The listing builds one solid part. Answer for the finished solid, in the listing's coordinates (mm). A direction names the side the tool comes from. Round coordinates to 2 decimals unless told otherwise and drop trailing zeros. Loops run counter-clockwise (first coordinate to the right, second up) from the corner with the lowest first, then second, coordinate; pieces in that order, holes last. Notation, with made-up numbers: (12, -19) - (69, -19) arc R3 ccw to (69, -15) - close; hole circle Ø2 at (89.5, 1). An arc over 180 degrees is marked (long way). One line per item, written item: value.
```python
from build123d import *

# Parameters (mm, degrees)
BOSS_EXTRUDE1_DEPTH = 5
FILLET1_R           = 0.5


with BuildPart() as part:
    # Sketch1 → Boss-Extrude1 (new body)
    with BuildSketch(Plane.XY):
        with BuildLine():
            Line((-58.035421321, -29.898049549), (-52.781533871, -38.998049549))
            Line((-52.781533871, -38.998049549), (-47.781533871, -38.998049549))
            Line((-47.781533871, -38.998049549), (-50.93623441, -40.998049549))
            Line((-50.93623441, -40.998049549), (-53.93623441, -40.998049549))
            Line((-53.93623441, -40.998049549), (-59.767472129, -30.898049549))
            ThreePointArc((-59.767472129, -30.898049549), (-61.401962202, -24.798049549), (-59.767472129, -18.698049549))
            Line((-59.767472129, -18.698049549), (-53.93623441, -8.598049549))
            Line((-53.93623441, -8.598049549), (-51.291363981, -8.598049549))
            ThreePointArc((-51.291363981, -8.598049549), (-48.766460182, -4.985563469), (-44.583160049, -3.598049549))
            Line((-44.583160049, -3.598049549), (-44.583160049, -5.598049549))
            ThreePointArc((-44.583160049, -5.598049549), (-48.118693955, -7.062515643), (-49.583160049, -10.598049549))
            Line((-49.583160049, -10.598049549), (-52.781533871, -10.598049549))
            Line((-52.781533871, -10.598049549), (-58.035421321, -19.698049549))
            ThreePointArc((-58.035421321, -19.698049549), (-59.401962202, -24.798049549), (-58.035421321, -29.898049549))
        make_face()
    boss_extrude1 = extrude(amount=BOSS_EXTRUDE1_DEPTH)

    # Mirror1: Boss-Extrude1 across plane
    add(boss_extrude1.mirror(Plane(origin=(-44.583160049, -5.598049549, 5), x_dir=(0, 0, 1), z_dir=(-1, 0, 0))))

    # Fillet1
    fillet1_edges = [part.edges().sort_by_distance(p)[0] for p in [
        (-47.781533871, -38.998049549, 2.5),
        (-50.93623441, -40.998049549, 2.5),
        (-53.93623441, -40.998049549, 2.5),
        (-53.93623441, -8.598049549, 2.5),
        (-51.291363981, -8.598049549, 2.5),
        (-41.384786226, -38.998049549, 2.5),
        (-38.230085688, -40.998049549, 2.5),
        (-35.230085688, -40.998049549, 2.5),
        (-35.230085688, -8.598049549, 2.5),
        (-37.874956116, -8.598049549, 2.5),
    ]]
    fillet(fillet1_edges, radius=FILLET1_R)


solid = part.part
```
1) Each of these flat-tipped pins is pushed along its axis until it touches: pin 1 Ø10 at (x, y) = (-48, -28.5) entering from -Z; pin 2 Ø3 at (y, z) = (-30.5, 4) entering from +X; pin 3 Ø2 at (x, z) = (-35.5, 3.5) entering from +Y; pin 4 Ø2 at (y, z) = (-33, 1.5) entering from +X. Where does it stop, or does it pass through?
Final values:
pin 1: through
pin 2: x = -28.51
pin 3: y = -8.6
pin 4: x = -30.04
2) For faces 1 (the flat face through (-53, -8.598, 2)), 2 (the flat face through (-50.01, -40.41, 2.46)), 3 (the flat face through (-33.795, -15.084, 2.465)), determine the directions among +Z, -Z, +X, -X, +Y, -Y from which every point of the face is accessible in a straight line to the end or side of a thin tool.
Final values:
face 1: +Z, -Z, -X, +Y
face 2: +Z, -Z, -Y
face 3: +Z, -Z
3) A cutting plane is placed at A-A on y = -27. Give the vertices of the cut face in (x, z).
Final values:
outline: (-61.2, 0) - (-59.16, 0) - (-59.16, 5) - (-61.2, 5) - close; (-30, 0) - (-27.96, 0) - (-27.96, 5) - (-30, 5) - close
4) A cutting plane is placed at B-B on x = -33. Give the vertices of the cut face in (y, z).
Final values:
outline: (-37.14, 0) - (-33.14, 0) - (-33.14, 5) - (-37.14, 5) - close; (-16.46, 0) - (-12.46, 0) - (-12.46, 5) - (-16.46, 5) - close
5) Consider L1, parallel to X at y = -25, z = 4.35; L2, parallel to Y at x = -52.5, z = 2.6; L3, parallel to X at y = -37, z = 3. Determine where each line is inside the solid, lowest interval first.
Final values:
L1: -61.4 to -59.4, -29.77 to -27.77
L2: -41 to -39, -10.6 to -8.6
L3: -56.24 to -53.94, -35.23 to -32.92
6) A cutting plane is placed at C-C on x = -47. Give the vertices of the cut face in (y, z), and give its area (3 significant figures).
Final values:
outline: (-6.22, 0) - (-4.03, 0) - (-4.03, 5) - (-6.22, 5) - close
area: 11.0 mm2
7) For a pull along X with two mould halves and no side action, classify faces 4 (the flat face through (-37, -8.598, 2)), 5 (the cylindrical face through (-61.4, -24.9, 2.5)), 6 (the flat face through (-38, -10.598, 2)) as released by +X, released by -X, zero draft, split by the parting line, or undercut.
Final values:
face 4: zero draft
face 5: released by -X
face 6: undercut
